from build123d import *

# Parameters (mm, degrees)
SKETCH1_W           = 12.5
SKETCH1_H           = 2.5
BOSS_EXTRUDE1_DEPTH = 0.4
SKETCH1_3_W         = 13.3
SKETCH1_3_H         = 3.3
SKETCH1_3_W_2       = 12.5
SKETCH1_3_H_2       = 2.5
EXTRUDE_THIN1_DEPTH = 4.2
SKETCH2_W           = 13.3
SKETCH2_H           = 4.2
BOSS_EXTRUDE2_DEPTH = 4.5
CUT_EXTRUDE1_DEPTH  = 12.077116051
FILLET1_R           = 0.6


with BuildPart() as part:
    # Sketch1 → Boss-Extrude1 (new body)
    with BuildSketch(Plane.XY):
        Rectangle(SKETCH1_W, SKETCH1_H)
    extrude(amount=BOSS_EXTRUDE1_DEPTH)

    # Sketch1<3> → Extrude-Thin1 (add)
    with BuildSketch(Plane.XY):
        Rectangle(SKETCH1_3_W, SKETCH1_3_H)
        Rectangle(SKETCH1_3_W_2, SKETCH1_3_H_2, mode=Mode.SUBTRACT)
    extrude(amount=EXTRUDE_THIN1_DEPTH)

    # Sketch2 → Boss-Extrude2 (add)
    with BuildSketch(Plane.XZ.offset(1.65)):
        with Locations((0, 2.1)):
            Rectangle(SKETCH2_W, SKETCH2_H)
    extrude(amount=BOSS_EXTRUDE2_DEPTH)

    # Sketch3 → Cut-Extrude1 (cut, through all)
    with BuildSketch(Plane(origin=(0, 1.65, 0), x_dir=(1, 0, 0), z_dir=(0, 1, 0))):
        with BuildLine():
            Line((1.15, -1.733499425), (1.15, -2.654986585))
            ThreePointArc((1.15, -2.654986585), (0, -3.804986585), (-1.15, -2.654986585))
            Line((-1.15, -2.654986585), (-1.15, -1.733499425))
            ThreePointArc((-1.15, -1.733499425), (0, -0.583499425), (1.15, -1.733499425))
        make_face()
    extrude(amount=-CUT_EXTRUDE1_DEPTH, mode=Mode.SUBTRACT)

    # Fillet1
    fillet1_edges = [part.edges().sort_by_distance(p)[0] for p in [
        (-6.65, 1.65, 2.1),
        (6.65, 1.65, 2.1),
        (-6.65, -6.15, 2.1),
        (6.65, -6.15, 2.1),
    ]]
    fillet(fillet1_edges, radius=FILLET1_R)


solid = part.part
Work out the finished part from the listing and answer in its coordinate system (mm). A direction names the side the tool comes from. Round coordinates to 2 decimals unless told otherwise and drop trailing zeros. Write each loop counter-clockwise with the first axis right and the second up, starting at its lowest first coordinate (ties: lowest second). Pieces come first, ordered by that corner, then holes. Notation, with made-up numbers: (57.25, 23) - (94.25, 23) arc R8 cw to (94.25, 36) - close; hole circle Ø7 at (52.25, -13). An arc over 180 degrees is marked (long way). Answer in a Markdown table with one row per item. Add a question column.
1. A cutting plane is placed at D-D, the plane x = -2.75. Determine the outline of the cut face in (y, z), and give its area (3 significant figures).
2. A cutting plane is placed at C-C, the plane y = -2.75. Determine the outline of the cut face in (x, z), and give its area (3 significant figures).
3. Find the intervals of material crossed by line 1 along X through (y, z) = (-0.75, 0.5); line 2 along X through (y, z) = (-2, 2.45); line 3 along Y through (x, z) = (0.5, 3.8), in increasing order. Write a range as from..to.
4. Given pin 1 (2 mm diameter, centred on x = -2, y = 0, fed in from +Z), flat-ended and moving along its own axis, determine where the tip first touches the part or whether it passes through.
5. The mould has two halves that part along Z. Classify faces 4 (the flat face through (1.301, -1.25, 2.273)), 5 (the flat face through (-1.15, -4, 2)), 6 (the flat face through (0, -3, 4.2)): +Z half, -Z half, draft (parallel to the pull), parting line (faces both ways), or undercut.
6. For faces 1 (the cylindrical face through (-0.025, 1.453, 0.584)), 2 (the flat face through (-1.4, 1.65, 2.1)), 3 (the flat face through (1.301, 1.25, 2.273)), determine the directions among +Z, -Z, +X, -X, +Y, -Y from which every point of the face is accessible in a straight line to the end or side of a thin tool.
7. A cutting plane is placed at A-A, the plane x = 0. Determine the outline of the cut face in (y, z), and give its area (3 significant figures).
8. A cutting plane is placed at B-B, the plane z = 3.5. Determine the outline of the cut face in (x, y), and give its area (3 significant figures).
Worked out:
| question | item | result |
|---|---|---|
| 1 | outline | (-6.15, 0) - (1.65, 0) - (1.65, 4.2) - (1.25, 4.2) - (1.25, 0.4) - (-1.25, 0.4) - (-1.25, 4.2) - (-6.15, 4.2) - close |
| 1 | area | 23.3 mm^2 |
| 2 | outline | (-6.65, 0) - (6.65, 0) - (6.65, 4.2) - (-6.65, 4.2) - close; hole (-1.15, 1.73) arc R1.15 ccw to (1.15, 1.73) - (1.15, 2.65) arc R1.15 ccw to (-1.15, 2.65) - close |
| 2 | area | 49.6 mm^2 |
| 3 | line 1 | -6.65..-6.25, 6.25..6.65 |
| 3 | line 2 | -6.65..-1.15, 1.15..6.65 |
| 3 | line 3 | -6.15..-1.25, 1.25..1.65 |
| 4 | pin 1 | z = 0.4 |
| 5 | face 4 | draft |
| 5 | face 5 | undercut |
| 5 | face 6 | +Z half |
| 6 | face 1 | +Y, -Y |
| 6 | face 2 | +Z, -Z, +X, -X, +Y |
| 6 | face 3 | +Z |
| 7 | outline | (-6.15, 0) - (1.65, 0) - (1.65, 0.58) - (1.25, 0.58) - (1.25, 0.4) - (-1.25, 0.4) - (-1.25, 0.58) - (-6.15, 0.58) - close; (-6.15, 3.8) - (-1.25, 3.8) - (-1.25, 4.2) - (-6.15, 4.2) - close; (1.25, 3.8) - (1.65, 3.8) - (1.65, 4.2) - (1.25, 4.2) - close |
| 7 | area | 6.19 mm^2 |
| 8 | outline | (-6.65, -5.55) arc R0.6 ccw to (-6.05, -6.15) - (-0.78, -6.15) - (-0.78, -1.25) - (-6.25, -1.25) - (-6.25, 1.25) - (-0.78, 1.25) - (-0.78, 1.65) - (-6.05, 1.65) arc R0.6 ccw to (-6.65, 1.05) - close; (0.78, -6.15) - (6.05, -6.15) arc R0.6 ccw to (6.65, -5.55) - (6.65, 1.05) arc R0.6 ccw to (6.05, 1.65) - (0.78, 1.65) - (0.78, 1.25) - (6.25, 1.25) - (6.25, -1.25) - (0.78, -1.25) - close |
| 8 | area | 63.9 mm^2 |
